Work out the finished part from the listing and answer in its coordinate system (mm). A direction names the side the tool comes from. Round coordinates to 2 decimals unless told otherwise and drop trailing zeros. Order: outer loops, then holes, each group sorted by start corner. A loop starts at its lowest first (then second) coordinate and runs counter-clockwise, first axis right, second up. Notation, with made-up numbers: M 13.25,30 L 52.25,30 A21 ccw 52.25,46 Z; hole C 59,25 d10. An arc over 180 degrees is marked long. Answer as a JSON object with one key per item and string values. Group by question number.
from build123d import *

# Parameters (mm, degrees)
BOSS_EXTRU_3_DEPTH      = 10
ENL_V_MAT_EXTRU_1_REACH = 56.156
ESQUISSE7_R             = 1
ENL_V_MAT_EXTRU_2_REACH = 53.855
ESQUISSE8_R             = 1.5
CONG_8_R                = 0.5


with BuildPart() as part:
    # Esquisse6 → Boss.-Extru.3 (new body)
    with BuildSketch(Plane.XY):
        Polygon((-32.5, -39.15), (-14.5, -39.15), (-14.5, 0), (14.5, 0), (14.5, -39.15), (32.5, -39.15), (32.5, -36.15), (17.5, -36.15), (17.5, 3), (-17.5, 3), (-17.5, -36.15), (-32.5, -36.15), align=None)
    extrude(amount=BOSS_EXTRU_3_DEPTH)

    # Esquisse7 → Enlèv. mat.-Extru.1 (cut, up to next)
    with BuildSketch(Plane(origin=(0, 3, 0), x_dir=(1, 0, 0), z_dir=(0, 1, 0)), mode=Mode.PRIVATE) as enl_v_mat_extru_1_sk1:
        with Locations(Location((-8.25, -5, 0), (0, 0, 180))):
            Circle(ESQUISSE7_R)
    enl_v_mat_extru_1_tool1 = extrude(enl_v_mat_extru_1_sk1.sketch, amount=-ENL_V_MAT_EXTRU_1_REACH, mode=Mode.PRIVATE) & part.part
    # Esquisse7 → Enlèv. mat.-Extru.1 (cut, up to next)
    with BuildSketch(Plane(origin=(0, 3, 0), x_dir=(1, 0, 0), z_dir=(0, 1, 0)), mode=Mode.PRIVATE) as enl_v_mat_extru_1_sk2:
        with Locations(Location((8.25, -5, 0), (0, 0, 180))):
            Circle(ESQUISSE7_R)
    enl_v_mat_extru_1_tool2 = extrude(enl_v_mat_extru_1_sk2.sketch, amount=-ENL_V_MAT_EXTRU_1_REACH, mode=Mode.PRIVATE) & part.part
    add(enl_v_mat_extru_1_tool1.solids().sort_by_distance((-8.25, 3, 5))[0], mode=Mode.SUBTRACT)
    add(enl_v_mat_extru_1_tool2.solids().sort_by_distance((8.25, 3, 5))[0], mode=Mode.SUBTRACT)

    # Esquisse8 → Enlèv. mat.-Extru.2 (cut, up to next)
    with BuildSketch(Plane(origin=(0, -36.15, 0), x_dir=(1, 0, 0), z_dir=(0, 1, 0)), mode=Mode.PRIVATE) as enl_v_mat_extru_2_sk1:
        with Locations(Location((27.5, -5, 0), (0, 0, 180))):
            Circle(ESQUISSE8_R)
    enl_v_mat_extru_2_tool1 = extrude(enl_v_mat_extru_2_sk1.sketch, amount=-ENL_V_MAT_EXTRU_2_REACH, mode=Mode.PRIVATE) & part.part
    # Esquisse8 → Enlèv. mat.-Extru.2 (cut, up to next)
    with BuildSketch(Plane(origin=(0, -36.15, 0), x_dir=(1, 0, 0), z_dir=(0, 1, 0)), mode=Mode.PRIVATE) as enl_v_mat_extru_2_sk2:
        with Locations(Location((-27.5, -5, 0), (0, 0, 180))):
            Circle(ESQUISSE8_R)
    enl_v_mat_extru_2_tool2 = extrude(enl_v_mat_extru_2_sk2.sketch, amount=-ENL_V_MAT_EXTRU_2_REACH, mode=Mode.PRIVATE) & part.part
    add(enl_v_mat_extru_2_tool1.solids().sort_by_distance((27.5, -36.15, 5))[0], mode=Mode.SUBTRACT)
    add(enl_v_mat_extru_2_tool2.solids().sort_by_distance((-27.5, -36.15, 5))[0], mode=Mode.SUBTRACT)

    # Congé8
    cong_8_edges = [part.edges().sort_by_distance(p)[0] for p in [
        (-32.5, -36.15, 5),
        (-17.5, -36.15, 5),
        (-17.5, 3, 5),
        (17.5, 3, 5),
        (17.5, -36.15, 5),
        (32.5, -36.15, 5),
    ]]
    fillet(cong_8_edges, radius=CONG_8_R)


solid = part.part
Item 1: Each of these flat-tipped pins is pushed along its axis until it touches: pin 1 (2 mm diameter, centred on y = -33.5, z = 2.5, fed in from -X); pin 2 (1.5 mm diameter, centred on y = -18, z = 1.5, fed in from +X). Where does it stop, or does it pass through?
Item 2: Find section A-A (x = 8.25). Give the vertices of the cut face in (y, z), and give its area (3 significant figures).
Item 3: Find section B-B (z = 5). Give the number of separate pieces and of enclosed holes in the cut face, and give its area (3 significant figures).
Item 4: The mould has two halves that part along Z. Classify faces 4 (the flat face through (-15, -16, 10)), 5 (the flat face through (0, 0, 5)), 6 (the cylindrical face through (-26, -38, 5)): +Z half, -Z half, draft (parallel to the pull), parting line (faces both ways), or undercut.
Item 5: Find section C-C (y = -13.5). Give the vertices of the cut face in (x, z), and give its area (3 significant figures).
Item 6: Consider L1, parallel to X at y = -22, z = 1.25; L2, parallel to Z at x = -8.25, y = 0.85; L3, parallel to Y at x = -2.5, z = 1.75. Determine where each line is inside the solid, lowest interval first.
Item 7: Find section D-D (z = 9.25). Give the vertices of the cut face in (x, y), and give its area (3 significant figures).
Item 8: A tool of negligible diameter and unlimited length cuts with its end or side. For faces 1 (the flat face through (-14.5, -20, 5)), 2 (the flat face through (25, -36.15, 5)), 3 (the flat face through (-17.5, -16, 5)), from which of +Z, -Z, +X, -X, +Y, -Y can it reach the whole face along a straight path? Write none if from no direction.
Responses:
{
 "1": {"pin 1": "stops at x = -17.5", "pin 2": "stops at x = 17.5"},
 "2": {"outline": "M 0,0 L 3,0 L 3,4 L 0,4 Z; M 0,6 L 3,6 L 3,10 L 0,10 Z", "area": "24.0 mm^2"},
 "3": {"separate pieces": "5", "enclosed holes": "0", "area": "400 mm^2"},
 "4": {"face 4": "+Z half", "face 5": "draft", "face 6": "undercut"},
 "5": {"outline": "M -17.5,0 L -14.5,0 L -14.5,10 L -17.5,10 Z; M 14.5,0 L 17.5,0 L 17.5,10 L 14.5,10 Z", "area": "60.0 mm^2"},
 "6": {"L1": "x = -17.5 to -14.5, 14.5 to 17.5", "L2": "z = 0 to 4, 6 to 10", "L3": "y = 0 to 3"},
 "7": {"outline": "M -32.5,-39.15 L -14.5,-39.15 L -14.5,0 L 14.5,0 L 14.5,-39.15 L 32.5,-39.15 L 32.5,-36.65 A0.5 ccw 32,-36.15 L 18,-36.15 A0.5 cw 17.5,-35.65 L 17.5,2.5 A0.5 ccw 17,3 L -17,3 A0.5 ccw -17.5,2.5 L -17.5,-35.65 A0.5 cw -18,-36.15 L -32,-36.15 A0.5 ccw -32.5,-36.65 Z", "area": "430 mm^2"},
 "8": {"face 1": "+Z, -Z, -Y", "face 2": "+Z, -Z, +X, +Y", "face 3": "+Z, -Z, -X, +Y"}
}
